```python
from build123d import *

# Parameters (mm, degrees)
CUT_EXTRUDE2_DEPTH = 0.91


with BuildPart() as part:
    # Sketch10 → Revolve3 (revolve)
    with BuildSketch(Plane(origin=(0, 0, 0), x_dir=(0, 0, -1), z_dir=(1, 0, 0)), mode=Mode.PRIVATE) as revolve3_sk:
        Polygon((13, 1), (13.3, 0.7), (13.3, 0), (1.3, 0), (1.3, 1), align=None)
    revolve(revolve3_sk.sketch.rotate(Axis((0, 0, 0), (0, 0, -1)), 90), axis=Axis((0, 0, 0), (0, 0, -1)))

    # Sketch7 → Revolve2 (revolve)
    with BuildSketch(Plane(origin=(0, 0, 0), x_dir=(0, 0, -1), z_dir=(1, 0, 0)), mode=Mode.PRIVATE) as revolve2_sk:
        with BuildLine():
            Line((1.105, 1.75), (1.3, 1.75))
            Line((1.3, 1.75), (1.3, 0))
            Line((1.3, 0), (0, 0))
            Line((0, 0), (0, 1))
            ThreePointArc((0, 1), (0.479976957, 1.481850617), (1.105, 1.75))
        make_face()
    revolve(revolve2_sk.sketch.rotate(Axis((0, 0, 0), (0, 0, -1)), 180), axis=Axis((0, 0, 0), (0, 0, -1)))

    # Sketch5 → Cut-Extrude2 (cut)
    with BuildSketch(Plane.XY):
        Polygon((0.65, -0.375277675), (0.65, 0.375277675), (0, 0.75055535), (-0.65, 0.375277675), (-0.65, -0.375277675), (0, -0.75055535), align=None)
    extrude(amount=-CUT_EXTRUDE2_DEPTH, mode=Mode.SUBTRACT)

    # Cut-Extrude3 cone 1 section (through the dimple's axis) → Cut-Extrude3 (revolve, cut)
    with BuildSketch(Plane(origin=(0, 0, 0), x_dir=(0, -1, 0), z_dir=(1, 0, 0))):
        Polygon((0, 0), (0.75055535, 0), (0, 0.75055535), align=None)
    revolve(axis=Axis((0, 0, 0), (0, 0, -1)), mode=Mode.SUBTRACT)


with BuildPart() as body_2:
    # Split1: read off the stored shape, not the designer's step
    # Split1: the piece on the far side of the plane
    add(part.part)
    split(bisect_by=Plane.XY.offset(-1.3), keep=Keep.BOTTOM)


with BuildPart() as part_1:
    add(part.part)

    # Split1
    split(bisect_by=Plane.XY.offset(-1.3), keep=Keep.TOP)


with BuildPart() as body_2_1:
    add(body_2.part)

    # Boss-Extrude1: read off the stored shape, not the designer's step
    # Boss-Extrude1: union part
    add(part_1.part)


solid = body_2_1.part
```
Verification items for the finished model (mm, model axes). Give positions to 0.01 mm unless a question says otherwise; leave off trailing zeros. Loops run counter-clockwise (first coordinate to the right, second up) from the corner with the lowest first, then second, coordinate; pieces in that order, holes last.
1. Thickness scan on line 1 (Z direction, x = 0.5, y = -0.2); line 2 (Y direction, x = 0, z = -8.5); line 3 (Y direction, x = 0.7, z = -4.5). Record the ranges inside material, lowest first.
2. Section check C-C, the plane x = -1.15. Enter the section's corners in (y, z) (3 decimals), then the cut area to 3 significant figures.
3. Section check A-A, the plane y = 0. Enter the section's corners in (x, z) (3 decimals).
4. Go/stop test with flat-tipped pins: pin 1 Ø0.8 at (y, z) = (0, -0.5) entering from +X; pin 2 Ø1 at (x, z) = (-1, -6) entering from +Y; pin 3 Ø2 at (y, z) = (0.5, -2.5) entering from -X. Record where each tip stops, or that it passes through.
5. Section check B-B, the plane z = -3.5. Enter the section's corners in (x, y).
6. Mould release check, pull along Y, two halves, no side actions. Record for faces 1 (the flat face through (0, 0, -0.91)), 2 (the flat face through (1, -1, -1.3)), 3 (the cylindrical face through (0, 1, -7)): released by +Y, released by -Y, zero draft, split by the parting line, or undercut.
Geometry says:
1. line 1: z = -13.3 to -0.91
1. line 2: y = -1 to 1
1. line 3: y = -0.71 to 0.71
2. outline: (-1.319, -1.3) - (1.319, -1.3) - (1.319, -1.105) arc R1.373 ccw to (-1.319, -1.105) - close
2. area: 2.44 mm2
3. outline: (-1.75, -1.3) - (-1, -1.3) - (-1, -13) - (-0.7, -13.3) - (0.7, -13.3) - (1, -13) - (1, -1.3) - (1.75, -1.3) - (1.75, -1.105) arc R1.791 ccw to (1, 0) - (0.751, 0) - (0.65, -0.101) - (0.65, -0.91) - (-0.65, -0.91) - (-0.65, -0.101) - (-0.751, 0) - (-1, 0) arc R1.791 ccw to (-1.75, -1.105) - close
4. pin 1: stops at x = 1.69
4. pin 2: stops at y = 0.87
4. pin 3: stops at x = -1
5. outline: circle Ø2 at (0, 0)
6. face 1: undercut
6. face 2: zero draft
6. face 3: split by the parting line
